```python
from build123d import *

# Parameters (mm, degrees)
SKETCH1_R           = 4.7625
BOSS_EXTRUDE2_DEPTH = 14


with BuildPart() as part:
    # Sketch1 → Boss-Extrude2 (new body)
    with BuildSketch(Plane(origin=(0, 0, 0), x_dir=(1, 0, 0), z_dir=(0, 1, 0))):
        Polygon((0, 300), (400, 300), (200, 0), (0, 0), (-200, 0), (-400, 300), align=None)
        with Locations(Location((0, 293, 0), (0, 0, 270))):
            Circle(SKETCH1_R, mode=Mode.SUBTRACT)
        with Locations(Location((0, 7, 0), (0, 0, 270))):
            Circle(SKETCH1_R, mode=Mode.SUBTRACT)
        with Locations(Location((384.258956968, 293, 0), (0, 0, 270))):
            Circle(SKETCH1_R, mode=Mode.SUBTRACT)
        with Locations(Location((-384.258956968, 293, 0), (0, 0, 90))):
            Circle(SKETCH1_R, mode=Mode.SUBTRACT)
        with Locations(Location((-195.793523512, 7, 0), (0, 0, 270))):
            Circle(SKETCH1_R, mode=Mode.SUBTRACT)
        with Locations(Location((195.793523512, 7, 0), (0, 0, 90))):
            Circle(SKETCH1_R, mode=Mode.SUBTRACT)
        Polygon((7, 14), (7, 266.380570536), (175.253713691, 14), align=None, mode=Mode.SUBTRACT)
        Polygon((10.746286309, 286), (373.840760715, 286), (190.836035912, 15.865375596), align=None, mode=Mode.SUBTRACT)
        Polygon((-190.947369666, 15.698374965), (-10.746286309, 286), (-368.994606868, 286), align=None, mode=Mode.SUBTRACT)
        Polygon((-175.253713691, 14), (-7, 266.380570536), (-7, 14), align=None, mode=Mode.SUBTRACT)
    extrude(amount=BOSS_EXTRUDE2_DEPTH)


solid = part.part
```
Input: part model. Units: mm. Frame: model coordinates. A direction names the side the tool comes from. Coordinates: 2 decimals unless noted, no trailing zeros. Loops run counter-clockwise (first coordinate to the right, second up) from the corner with the lowest first, then second, coordinate; pieces in that order, holes last. Notation, with made-up numbers: (76.5, 20.25) - (121.5, 20.25) arc R16 ccw to (121.5, 46.25) - close; hole circle Ø10 at (9.5, -6). An arc over 180 degrees is marked (long way). Answer in a Markdown table with one row per item.
(1) Pin query (flat end, axial travel): P1, Ø5.5, axis at x = -384.26, z = -293, coming from the -Y side; P2, Ø4, axis at y = 4.5, z = -202.5, coming from the -X side; P3, Ø6, axis at x = 296.5, y = 4.5, coming from the +Z side; P4, Ø8, axis at y = 3, z = -240, coming from the +X side. Return the tip coordinate at first contact, or that it passes through.
Model answer:
| item | result |
|---|---|
| P1 | passes through |
| P2 | stops at x = -336.33 |
| P3 | stops at z = -140.25 |
| P4 | stops at x = 362.67 |
(2) Cut plane C-C on y = 7.25. Count the separate pieces of the cut face and the enclosed holes in it, plus the area to 3 significant figures.
Model answer:
| item | result |
|---|---|
| separate pieces | 1 |
| enclosed holes | 10 |
| area | 39,600 mm² |
(3) Set-up query: faces 1 (the face through (-187, 7, -286)), 2 (the face through (2, 14, -162)). Return all of +Z, -Z, +X, -X, +Y, -Y with unobstructed straight access to the full face (end or side cutting, diameter ignored); none if empty.
Model answer:
| item | result |
|---|---|
| face 1 | +Y, -Y |
| face 2 | +Z, -Z, +X, -X, +Y |
(4) Cut plane D-D on z = -257. Output: boundary loops of the cut face in (x, y).
Model answer:
| item | result |
|---|---|
| outline | (-371.33, 0) - (-349.89, 0) - (-349.89, 14) - (-371.33, 14) - close; (-30.08, 0) - (-13.25, 0) - (-13.25, 14) - (-30.08, 14) - close; (-7, 0) - (7, 0) - (7, 14) - (-7, 14) - close; (13.25, 0) - (30.08, 0) - (30.08, 14) - (13.25, 14) - close; (354.19, 0) - (371.33, 0) - (371.33, 14) - (354.19, 14) - close |
(5) Cut plane A-A on z = -68. Output: boundary loops of the cut face in (x, y).
Model answer:
| item | result |
|---|---|
| outline | (-245.33, 0) - (-225.4, 0) - (-225.4, 14) - (-245.33, 14) - close; (-156.08, 0) - (-139.25, 0) - (-139.25, 14) - (-156.08, 14) - close; (-7, 0) - (7, 0) - (7, 14) - (-7, 14) - close; (139.25, 0) - (156.08, 0) - (156.08, 14) - (139.25, 14) - close; (226.16, 0) - (245.33, 0) - (245.33, 14) - (226.16, 14) - close |
(6) Material intervals for L1, parallel to X at y = 1, z = -81; L2, parallel to X at y = 8.25, z = -188; L3, parallel to X at y = 8.75, z = -293, sorted ascending. Write a range as from..to.
Model answer:
| item | result |
|---|---|
| L1 | x = -254..-233.96, -147.41..-130.59, -7..7, 130.59..147.41, 234.96..254 |
| L2 | x = -325.33..-304.44, -76.08..-59.25, -7..7, 59.25..76.08, 307.45..325.33 |
| L3 | x = -395.33..-389.02, -379.5..-4.76, 4.76..379.5, 389.02..395.33 |
(7) Cut plane B-B on x = 319. Output: boundary loops of the cut face in (y, z), plus the area to 3 significant figures.
Model answer:
| item | result |
|---|---|
| outline | (0, -300) - (14, -300) - (14, -286) - (0, -286) - close; (0, -205.05) - (14, -205.05) - (14, -178.5) - (0, -178.5) - close |
| area | 568 mm² |
(8) Mould query, pull axis Z, two halves, no side actions, for faces 3 (the face through (-281.217, 6.902, -152.741)), 4 (the face through (6, 7, -300)), 5 (the face through (-3, 7, 0)). Classes: pulls with the +Z half, pulls with the -Z half, needs draft (parallel to the pull), parting line crosses it, or undercut.
Model answer:
| item | result |
|---|---|
| face 3 | undercut |
| face 4 | pulls with the -Z half |
| face 5 | pulls with the +Z half |
